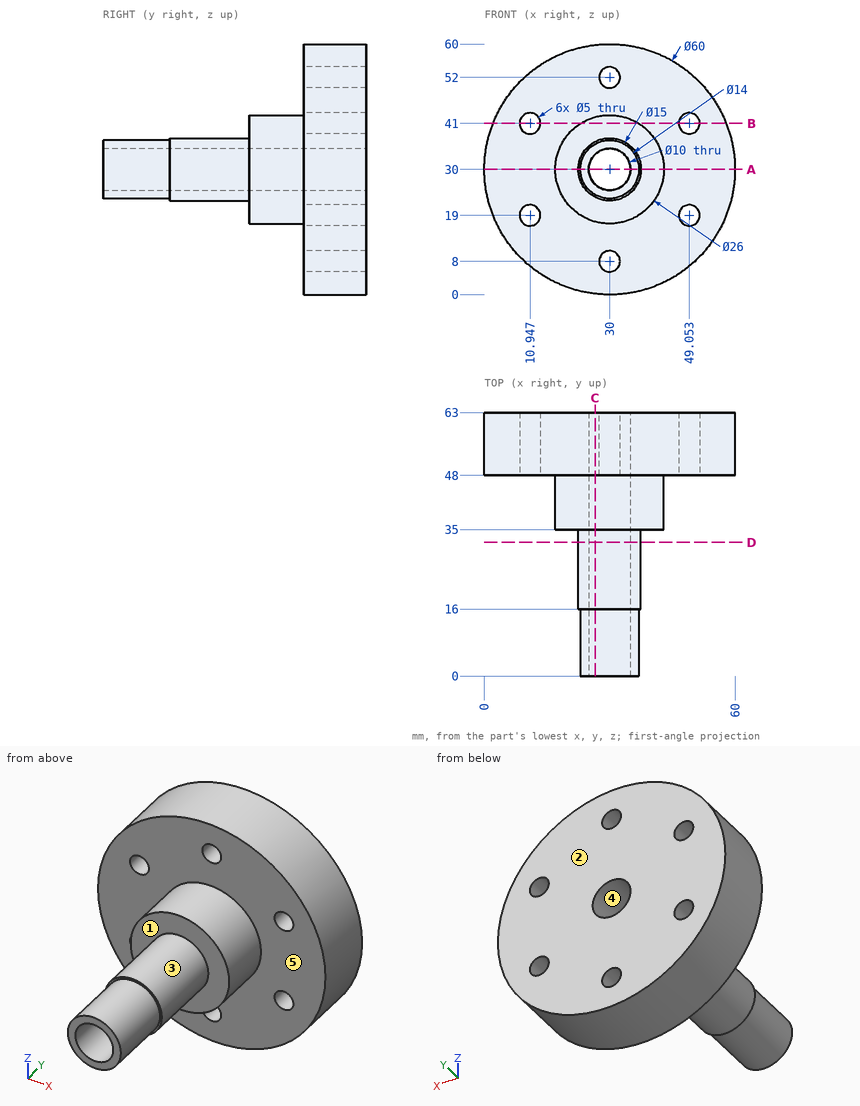
Here's the drawing with two shaded views (mm, measured from the low corner). I have some questions. A direction names the side the tool comes from. Give positions to 0.01 mm unless a question says otherwise; leave off trailing zeros. Loops run counter-clockwise (first coordinate to the right, second up) from the corner with the lowest first, then second, coordinate; pieces in that order, holes last. Notation, with made-up numbers: (58.5, 27.5) -> (106.5, 27.5) arc R29 ccw to (106.5, 64.5) -> close; hole circle Ø2 at (-7.5, -30). An arc over 180 degrees is marked (long way). Use one line per item in the form item = value.
1) If we section it at B-B (z = 41): Please give me the cut outline in (x, y).
Answers:
outline = (2.09, 48) -> (8.45, 48) -> (8.45, 63) -> (2.09, 63) -> close; (13.45, 48) -> (23.07, 48) -> (23.07, 35) -> (36.93, 35) -> (36.93, 48) -> (46.55, 48) -> (46.55, 63) -> (13.45, 63) -> close; (51.55, 48) -> (57.91, 48) -> (57.91, 63) -> (51.55, 63) -> close
2) We'd pull the mould along X, two halves only. Please class the marked faces 3, 4 and 5: released by +X, released by -X, zero draft, split by the parting line, or undercut.
Answers:
face_3 = split by the parting line
face_4 = undercut
face_5 = zero draft
3) Will these pins go through, and if not, where does the flat tip stop? pin 1 (8 mm diameter, centred on x = 8.5, y = 55.5, fed in from -Z); pin 2 (6 mm diameter, centred on x = 49.05, z = 19, fed in from -Y); pin 3 (4 mm diameter, centred on y = 44, z = 39, fed in from -X) (1 decimal).
Answers:
pin_1 = 5.63
pin_2 = 48
pin_3 = 19
4) If we section it at D-D (y = 32): Please give me the cut outline in (x, z).
Answers:
outline = circle Ø15 at (30, 30); hole circle Ø10 at (30, 30)
5) If we section it at A-A (z = 30): Please give me the cut outline in (x, y), plus the area to 3 significant figures.
Answers:
outline = (0, 48) -> (17, 48) -> (17, 35) -> (22.5, 35) -> (22.5, 16) -> (23, 16) -> (23, 0) -> (25, 0) -> (25, 63) -> (0, 63) -> close; (35, 0) -> (37, 0) -> (37, 16) -> (37.5, 16) -> (37.5, 35) -> (43, 35) -> (43, 48) -> (60, 48) -> (60, 63) -> (35, 63) -> close
area = 1,120 mm²
6) I need wall thicknesses on line 1 along X through (y, z) = (29.5, 30); line 2 along Z through (x, y) = (30, 56); line 3 along Y through (x, z) = (26, 52.5). Which ranges of each line are inside material? Lowest first, please.
Answers:
line_1 = 22.5 to 25, 35 to 37.5
line_2 = 0 to 5.5, 10.5 to 25, 35 to 49.5, 54.5 to 60
line_3 = 48 to 63
7) If we section it at C-C (x = 26.5): Please give me the cut outline in (y, z) (1 decimal), plus the area to 3 significant figures.
Answers:
outline = (0, 23.9) -> (16, 23.9) -> (16, 23.4) -> (35, 23.4) -> (35, 17.5) -> (48, 17.5) -> (48, 0.2) -> (63, 0.2) -> (63, 26.4) -> (0, 26.4) -> close; (0, 33.6) -> (63, 33.6) -> (63, 59.8) -> (48, 59.8) -> (48, 42.5) -> (35, 42.5) -> (35, 36.6) -> (16, 36.6) -> (16, 36.1) -> (0, 36.1) -> close
area = 1,220 mm²
8) For the marked faces 1 and 2, which set-ups out of +Z, -Z, +X, -X, +Y, -Y let a thin tool reach every point of the face, with its end or its side?
Answers:
face_1 = -Y
face_2 = +Z, -Z, +X, -X, +Y
